Here's the drawing with two shaded views (mm, measured from the low corner). I have some questions. Round coordinates to 2 decimals unless told otherwise and drop trailing zeros. Loops run counter-clockwise (first coordinate to the right, second up) from the corner with the lowest first, then second, coordinate; pieces in that order, holes last. Notation, with made-up numbers: (86, 16.25) - (112, 16.25) arc R23 ccw to (112, 26.25) - close; hole circle Ø1 at (21.25, -12). An arc over 180 degrees is marked (long way). Answer as CSV lines item,"result".
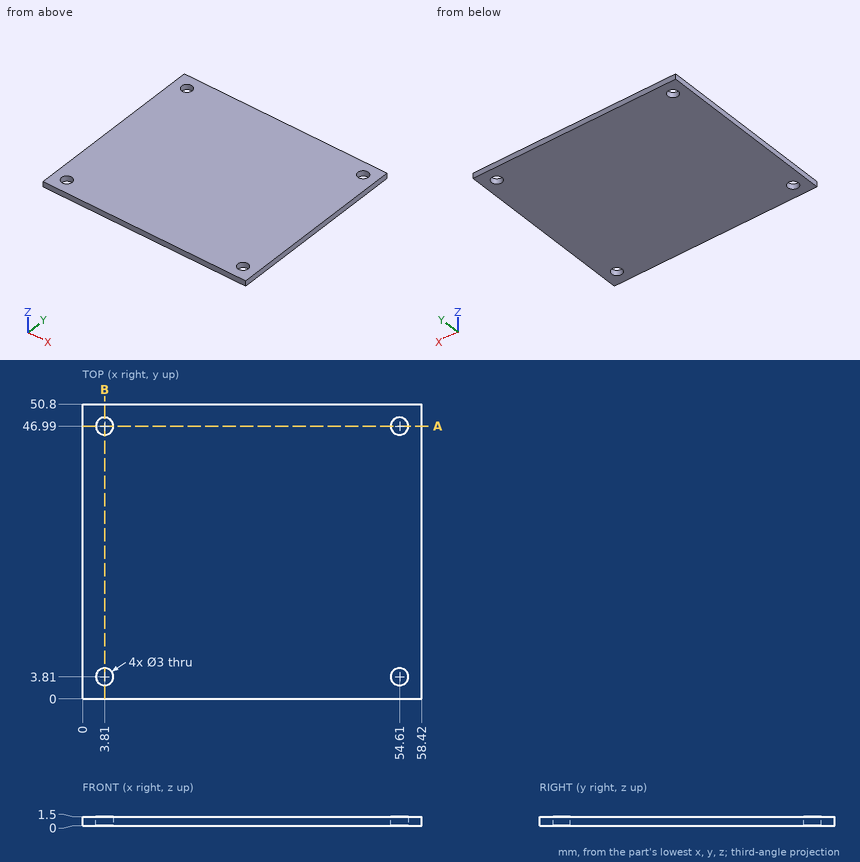
Q1. Imagine slicing it at B-B (x = 3.81). Write out the boundary of the cut face in (y, z), then the cut area to 3 significant figures.
Checks:
outline,"(0, 0) - (2.31, 0) - (2.31, 1.5) - (0, 1.5) - close; (5.31, 0) - (45.49, 0) - (45.49, 1.5) - (5.31, 1.5) - close; (48.49, 0) - (50.8, 0) - (50.8, 1.5) - (48.49, 1.5) - close"
area,"67.2 mm²"
Q2. Imagine slicing it at A-A (y = 46.99). Write out the boundary of the cut face in (x, z).
Checks:
outline,"(0, 0) - (2.31, 0) - (2.31, 1.5) - (0, 1.5) - close; (5.31, 0) - (53.11, 0) - (53.11, 1.5) - (5.31, 1.5) - close; (56.11, 0) - (58.42, 0) - (58.42, 1.5) - (56.11, 1.5) - close"
Q3. If I drill on line 1 along Y through (x, z) = (3.81, 0.55); line 2 along X through (y, z) = (46.99, 0.8); line 3 along X through (y, z) = (3, 0.9), over which ranges is the centre line in solid material (lowest first)? Write a range as [from, to].
Checks:
line 1,"[0, 2.31], [5.31, 45.49], [48.49, 50.8]"
line 2,"[0, 2.31], [5.31, 53.11], [56.11, 58.42]"
line 3,"[0, 2.55], [5.07, 53.35], [55.87, 58.42]"
